Read the model definition and answer for the solid it produces. Units are mm, in the model's axes. A direction names the side the tool comes from. Coordinates: 2 decimals unless noted, no trailing zeros. Order: outer loops, then holes, each group sorted by start corner. A loop starts at its lowest first (then second) coordinate and runs counter-clockwise, first axis right, second up. Notation, with made-up numbers: (14, -19) - (60, -19) arc R10 cw to (60, -9) - close; hole circle Ø7 at (15, -34.75). An arc over 180 degrees is marked (long way). Use one line per item in the form item = value. Start each with the question number.
from build123d import *

# Parameters (mm, degrees)
SKETCH1_R                = 2.5
BOSS_EXTRUDE4_DEPTH      = 5
BOSS_EXTRUDE5_DEPTH      = 17
BOSS_EXTRUDE5_DEPTH_BACK = 5
BOSS_EXTRUDE6_DEPTH      = 17
BOSS_EXTRUDE6_DEPTH_BACK = 5
SKETCH3_R                = 0.5
CUT_EXTRUDE4_DEPTH       = 17
SKETCH6_R                = 0.995072339
CUT_EXTRUDE5_DEPTH       = 25
SKETCH10_W               = 12.090214455
SKETCH10_H               = 12.735025893
SKETCH10_W_2             = 13.963890252
SKETCH10_H_2             = 14.708631066
BOSS_EXTRUDE8_DEPTH      = 5
SKETCH11_W               = 13.591519846
SKETCH11_H               = 14.150075456
BOSS_EXTRUDE9_DEPTH      = 5
SKETCH15_R               = 2.5
CUT_EXTRUDE7_DEPTH       = 7
SKETCH14_R               = 2.5
CUT_EXTRUDE8_DEPTH       = 7


with BuildPart() as part:
    # Sketch1 → Boss-Extrude4 (new body)
    with BuildSketch(Plane(origin=(0, 0, 0), x_dir=(1, 0, 0), z_dir=(0, 1, 0))):
        Polygon((-68.817127072, 2.747237569), (-0.817127072, 2.747237569), (-0.817127072, -65.252762431), (-17.817127072, -65.252762431), (-68.817127072, -14.252762431), align=None)
        with Locations((-9.317127072, -5.752762431)):
            Circle(SKETCH1_R, mode=Mode.SUBTRACT)
        with Locations((-26.317127072, -5.752762431)):
            Circle(SKETCH1_R, mode=Mode.SUBTRACT)
        with Locations((-43.317127072, -5.752762431)):
            Circle(SKETCH1_R, mode=Mode.SUBTRACT)
        with Locations((-60.317127072, -5.752762431)):
            Circle(SKETCH1_R, mode=Mode.SUBTRACT)
        with Locations((-9.317127072, -22.752762431)):
            Circle(SKETCH1_R, mode=Mode.SUBTRACT)
        with Locations((-9.317127072, -39.752762431)):
            Circle(SKETCH1_R, mode=Mode.SUBTRACT)
        with Locations((-9.317127072, -56.752762431)):
            Circle(SKETCH1_R, mode=Mode.SUBTRACT)
        with Locations((-37.306719432, -33.742354791)):
            Circle(SKETCH1_R, mode=Mode.SUBTRACT)
        Polygon((-17.817127072, -14.252762431), (-44.775496511, -14.252762431), (-17.817127072, -41.211131871), align=None, mode=Mode.SUBTRACT)
    extrude(amount=BOSS_EXTRUDE4_DEPTH)

    # Sketch2 → Boss-Extrude5 (add, two sides)
    with BuildSketch(Plane(origin=(0, 5, 0), x_dir=(1, 0, 0), z_dir=(0, 1, 0))) as boss_extrude5_sk:
        Polygon((-17.817127072, -14.252762431), (-44.775496511, -14.252762431), (-17.817127072, -41.211131871), align=None)
    extrude(amount=BOSS_EXTRUDE5_DEPTH)
    extrude(boss_extrude5_sk.sketch, amount=-BOSS_EXTRUDE5_DEPTH_BACK)

    # Sketch4 → Boss-Extrude6 (add, two sides)
    with BuildSketch(Plane(origin=(0, 5, 0), x_dir=(1, 0, 0), z_dir=(0, 1, 0))) as boss_extrude6_sk:
        Polygon((-0.817127072, -31.252762431), (-0.817127072, 2.747237569), (-34.817127072, 2.747237569), (-34.817127072, -14.252762431), (-17.817127072, -14.252762431), (-17.817127072, -31.252762431), align=None)
    extrude(amount=BOSS_EXTRUDE6_DEPTH)
    extrude(boss_extrude6_sk.sketch, amount=-BOSS_EXTRUDE6_DEPTH_BACK)

    # Sketch3 → Cut-Extrude4 (cut)
    with BuildSketch(Plane(origin=(-29.514129471, 0, 29.514129471), x_dir=(0.707106781, 0, 0.707106781), z_dir=(-0.707106781, 0, 0.707106781))):
        with Locations((-2.520386408, 18.449747468)):
            Circle(SKETCH3_R)
        with Locations((2.42936106, 13.5)):
            Circle(SKETCH3_R)
        with Locations((-2.520386408, 8.550252532)):
            Circle(SKETCH3_R)
        with Locations((-7.463225234, 13.549854817)):
            Circle(SKETCH3_R)
        Polygon((-7.470133876, 13.5), (-2.520386408, 18.449747468), (2.42936106, 13.5), (-2.520386408, 8.550252532), align=None)
    extrude(amount=-CUT_EXTRUDE4_DEPTH, mode=Mode.SUBTRACT)

    # Sketch6 → Cut-Extrude5 (cut)
    with BuildSketch(Plane(origin=(0, 22, 0), x_dir=(1, 0, 0), z_dir=(0, 1, 0))):
        with Locations((-31.26687454, -5.752762431)):
            Circle(SKETCH6_R)
        with Locations((-26.313804451, -10.748453884)):
            Circle(SKETCH6_R)
        with Locations((-21.367379604, -5.752762431)):
            Circle(SKETCH6_R)
        with Locations((-26.317127072, -0.803014963)):
            Circle(SKETCH6_R)
        Polygon((-31.26687454, -5.752762431), (-26.317127072, -10.702509899), (-21.367379604, -5.752762431), (-26.317127072, -0.803014963), align=None)
        with Locations((-14.26687454, -5.752762431)):
            Circle(SKETCH6_R)
        with Locations((-9.313804451, -10.748453884)):
            Circle(SKETCH6_R)
        with Locations((-4.367379604, -5.752762431)):
            Circle(SKETCH6_R)
        with Locations((-9.317127072, -0.803014963)):
            Circle(SKETCH6_R)
        Polygon((-14.26687454, -5.752762431), (-9.317127072, -10.702509899), (-4.367379604, -5.752762431), (-9.317127072, -0.803014963), align=None)
        with Locations((-14.26687454, -22.752762431)):
            Circle(SKETCH6_R)
        with Locations((-9.313804451, -27.748453884)):
            Circle(SKETCH6_R)
        with Locations((-4.367379604, -22.752762431)):
            Circle(SKETCH6_R)
        with Locations((-9.317127072, -17.803014963)):
            Circle(SKETCH6_R)
        Polygon((-14.26687454, -22.752762431), (-9.317127072, -27.702509899), (-4.367379604, -22.752762431), (-9.317127072, -17.803014963), align=None)
    extrude(amount=-CUT_EXTRUDE5_DEPTH, mode=Mode.SUBTRACT)

    # Sketch10 → Boss-Extrude8 (add)
    with BuildSketch(Plane.XZ):
        with Locations((-26.432881039, 5.808957337)):
            Rectangle(SKETCH10_W, SKETCH10_H)
        with Locations((-9.402846812, 23.47953019)):
            Rectangle(SKETCH10_W_2, SKETCH10_H_2)
    extrude(amount=-BOSS_EXTRUDE8_DEPTH)

    # Sketch11 → Boss-Extrude9 (add)
    with BuildSketch(Plane(origin=(0, 22, 0), x_dir=(1, 0, 0), z_dir=(0, 1, 0))):
        with Locations((-8.658105999, -5.978121074)):
            Rectangle(SKETCH11_W, SKETCH11_H)
    extrude(amount=-BOSS_EXTRUDE9_DEPTH)

    # Sketch15 → Cut-Extrude7 (cut)
    with BuildSketch(Plane(origin=(-0.817127072, 0, 0), x_dir=(0, 0, -1), z_dir=(1, 0, 0))):
        with Locations((-5.752762431, 13.5)):
            Circle(SKETCH15_R)
        with Locations((-22.752762431, 13.5)):
            Circle(SKETCH15_R)
    extrude(amount=-CUT_EXTRUDE7_DEPTH, mode=Mode.SUBTRACT)

    # Sketch14 → Cut-Extrude8 (cut)
    with BuildSketch(Plane(origin=(0, 0, -2.747237569), x_dir=(-1, 0, 0), z_dir=(0, 0, -1))):
        with Locations((26.317127072, 13.5)):
            Circle(SKETCH14_R)
        with Locations((9.317127072, 13.5)):
            Circle(SKETCH14_R)
    extrude(amount=-CUT_EXTRUDE8_DEPTH, mode=Mode.SUBTRACT)


solid = part.part
Q1. A cutting plane is placed at A-A (x = -37). Give the vertices of the cut face in (y, z).
Q2. Consider probe 1 along Z at (x, y) = (-6.5, 13.25); probe 2 along X at (y, z) = (18, 26.5); probe 3 along Z at (x, y) = (-23, 11). Determine where each line is inside the solid, lowest interval first.
Q3. Which of the six approach directions +Z, -Z, +X, -X, +Y, -Y give full straight-line access (tool end or side, diameter ignored) to faces 4 (the cylindrical face through (-9.345, 8.619, 11.743)), 5 (the flat face through (-23.599, 11.055, 23.577)), 6 (the cylindrical face through (-26.28, 8.15, -0.19)), 7 (the flat face through (-9, 13, 31.253)), 8 (the cylindrical face through (-62.815, 2.465, 5.643))?
Q4. For a pull along Y with two mould halves and no side action, classify faces 1 (the flat face through (-10, 17, 6)), 2 (the flat face through (-19.327, 13.576, 15.66)), 3 (the cylindrical face through (-26.28, 18.94, -0.19)) as +Y half, -Y half, draft (parallel to the pull), parting line (faces both ways), or undercut.
Q5. A cutting plane is placed at B-B (z = 46). Give the vertices of the cut face in (x, y).
Q6. Given P1, Ø4, axis at y = 13.5, z = 22.75, coming from the +X side; P2, Ø4, axis at x = -60.32, z = 5.75, coming from the -Y side; P3, Ø8.5, axis at y = 10.5, z = 7.5, coming from the -X side; P4, Ø6, axis at x = -44, y = 13.5, coming from the -Z side, each flat-ended and moving along its own axis, determine where each tip first touches the part or whether it passes through.
Result sheet:
q1.outline = (0, -2.75) - (5, -2.75) - (5, 14.25) - (22, 14.25) - (22, 22.03) - (5, 22.03) - (5, 31.26) - (0, 31.26) - close; (0, 36.22) - (5, 36.22) - (5, 46.07) - (0, 46.07) - close
q2.probe_1 = -2.75 to 3.27, 8.24 to 20.27, 25.24 to 31.25
q2.probe_2 = -32.53 to -30.7, -29.43 to -10.52, -8.11 to -0.82
q2.probe_3 = -2.75 to 4.12, 7.39 to 15.97, 22.9 to 36.03
q3.face_4 = -Y
q3.face_5 = none
q3.face_6 = +Y
q3.face_7 = +Z, +X, +Y
q3.face_8 = +Y, -Y
q4.face_1 = -Y half
q4.face_2 = undercut
q4.face_3 = draft
q5.outline = (-37.07, 0) - (-0.82, 0) - (-0.82, 5) - (-37.07, 5) - close
q6.P1 = -12.26
q6.P2 = through
q6.P3 = -34.82
q6.P4 = 14.25
